from build123d import *

# Parameters (mm, degrees)
F2_R     = 3.8487
F3_DEPTH = 50.8


with BuildPart() as f1:
    # F0 (on Top) → F1 (revolve)
    with BuildSketch(Plane.XY):
        Polygon((35.50566, 55.65488), (25.920112, 55.65488), (0, 0), (0, -44.308718), (4.988399, -44.308718), (4.988399, 0), align=None)
    revolve(axis=Axis((0, -22.154359, 0), (0, 1, 0)))

    # F2 (on face) → F3 (cut)
    with BuildSketch(Plane.XZ.offset(44.308718)):
        Circle(F2_R)
    extrude(amount=-F3_DEPTH, mode=Mode.SUBTRACT)


solid = f1.part
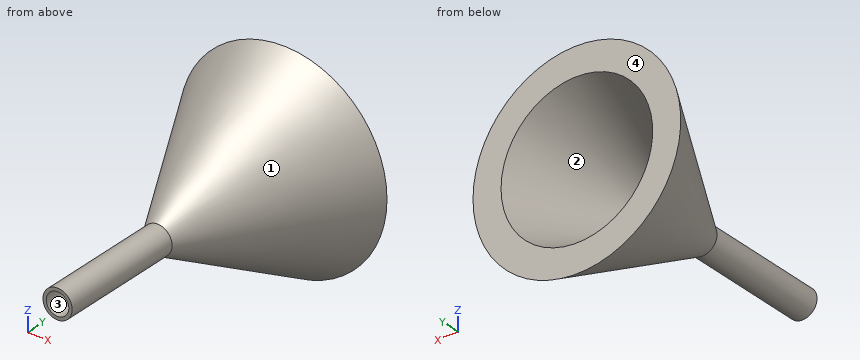
Could you check a few things on this model? Use its own coordinates, in mm. Face numbers are marked on the shaded views. Coordinates: 2 decimals unless noted, no trailing zeros. Order: outer loops, then holes, each group sorted by start corner. A loop starts at its lowest first (then second) coordinate and runs counter-clockwise, first axis right, second up. Notation, with made-up numbers: (59, 43.25) -> (115, 43.25) arc R20 cw to (115, 73.25) -> close; hole circle Ø10 at (28, -12.5). An arc over 180 degrees is marked (long way). One line per question, with ' | ' between items.
Q1. Imagine slicing it at C-C on y = 48. Please give me the cut outline in (x, z) (3 decimals), and give its area (3 significant figures).
Return value:
outline: circle Ø62.617 at (0, 0); hole circle Ø44.71 at (0, 0) | area: 1,510 mm²
Q2. Thinking about a two-plate mould opening in Z: for the marked faces 1, 2, 3 and 4, which applies, pulls with the +Z half, pulls with the -Z half, needs draft (parallel to the pull), parting line crosses it, or undercut?
Return value:
face 1: parting line crosses it | face 2: undercut | face 3: undercut | face 4: needs draft
Q3. Imagine slicing it at A-A on z = 0. Please give me the cut outline in (x, y), and give its area (3 significant figures).
Return value:
outline: (-35.51, 55.65) -> (-4.99, 0) -> (-4.99, -44.31) -> (-3.85, -44.31) -> (-3.85, 6.49) -> (-3.02, 6.49) -> (-25.92, 55.65) -> close; (3.02, 6.49) -> (3.85, 6.49) -> (3.85, -44.31) -> (4.99, -44.31) -> (4.99, 0) -> (35.51, 55.65) -> (25.92, 55.65) -> close | area: 882 mm²
Q4. If I drill on L1, parallel to Z at x = 0, y = -26; L2, parallel to Z at x = -17, y = 44.5; L3, parallel to X at y = 24.5, z = 7.5, over which ranges is the centre line in solid material (lowest first)?
Return value:
L1: -4.99 to -3.85, 3.85 to 4.99 | L2: -23.97 to -11.85, 11.85 to 23.97 | L3: -16.83 to -8.6, 8.6 to 16.83
Q5. Imagine slicing it at D-D on y = 29.5. Please give me the cut outline in (x, z).
Return value:
outline: circle Ø42.33 at (0, 0); hole circle Ø27.48 at (0, 0)
Q6. I'm going to push flat-ended pins straight in: P1, Ø10, axis at x = 5, y = 20, coming from the -Z side; P2, Ø2, axis at x = -6, z = 17.5, coming from the +Y side; P3, Ø12.5, axis at x = 0, z = 0, coming from the +Y side. Where does each tip first touch, or does it pass through?
Return value:
P1: z = -18.24 | P2: y = 41.87 | P3: y = 13.42
Q7. Imagine slicing it at B-B on x = 0. Please give me the cut outline in (y, z).
Return value:
outline: (-44.31, -4.99) -> (0, -4.99) -> (55.65, -35.51) -> (55.65, -25.92) -> (6.49, -3.02) -> (6.49, -3.85) -> (-44.31, -3.85) -> close; (-44.31, 3.85) -> (6.49, 3.85) -> (6.49, 3.02) -> (55.65, 25.92) -> (55.65, 35.51) -> (0, 4.99) -> (-44.31, 4.99) -> close
